Geometry: see drawing. Coordinates: mm, zero at the bounding-box minimum. A direction names the side the tool comes from. Round coordinates to 2 decimals unless told otherwise and drop trailing zeros. Order: outer loops, then holes, each group sorted by start corner. A loop starts at its lowest first (then second) coordinate and runs counter-clockwise, first axis right, second up. Notation, with made-up numbers: (-4.5, -15) - (41.5, -15) arc R19 ccw to (41.5, 15) - close; hole circle Ø5 at (89, -38). An arc over 180 degrees is marked (long way). Put each result on its own line as item: value. Start each with the question number.
1) Access query for the marked faces 1, 2 and 3. Directions: +Z, -Z, +X, -X, +Y, -Y. A direction counts if a zero-diameter tool reaches every point of the face in a straight line with its end or side. Return the directions, or none.
2) Contact query for flat-ended pins moving along their axis: P1, Ø6.5, axis at x = 22, y = 5, coming from the -Z side; P2, Ø4, axis at y = 8.5, z = 12.5, coming from the +X side. Output: stop coordinate, or through.
3) Section A-A on y = 25. Output: boundary loops of the cut face in (x, z).
4) Section B-B on x = 17. Output: boundary loops of the cut face in (y, z), then the cut area to 3 significant figures.
5) Line query: probe 1 along X at (y, z) = (28, 23.5); probe 2 along Y at (x, z) = (40.5, 13); probe 3 along Y at (x, z) = (10, 18.75). Output: solid intervals per line, ascending. Write a range as [from, to].
6) Section C-C on y = 2.5. Output: boundary loops of the cut face in (x, z).
7) Section D-D on x = 10. Output: boundary loops of the cut face in (y, z), then the cut area to 3 significant figures.
8) Mould query, pull axis X, two halves, no side actions, for the marked faces 4, 5 and 6. Classes: +X half, -X half, draft (parallel to the pull), parting line (faces both ways), or undercut.
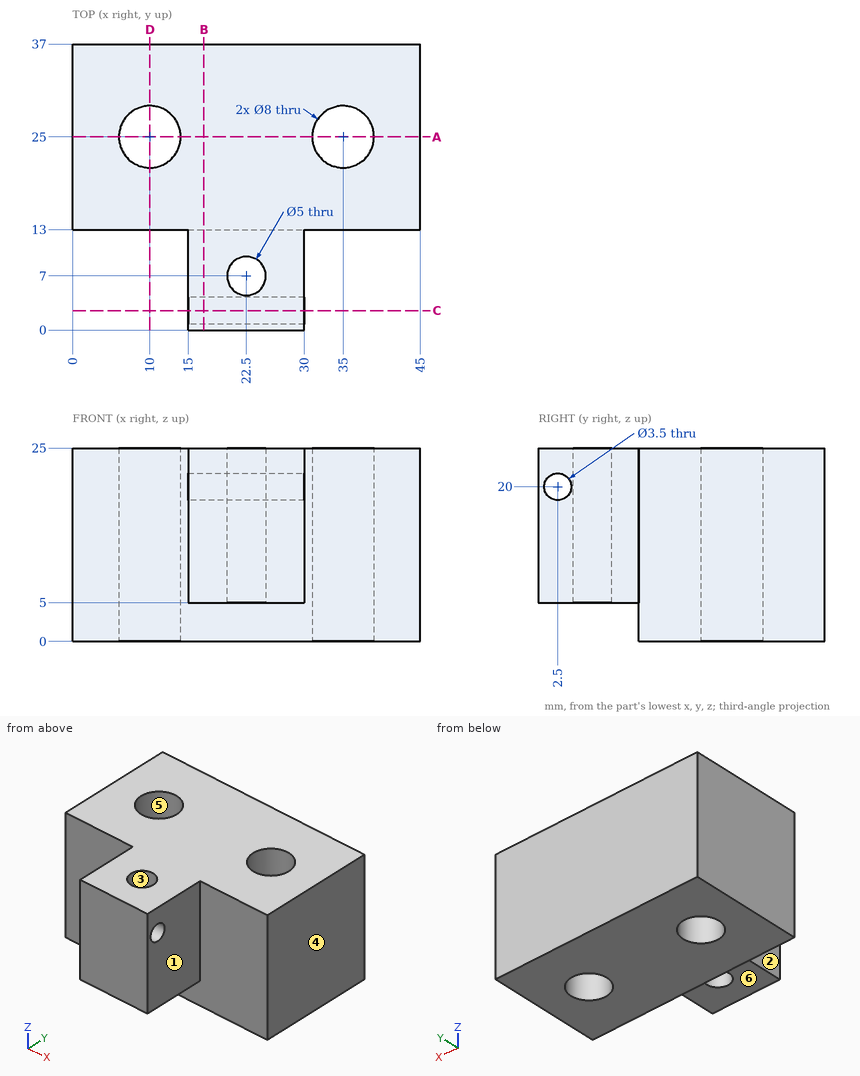
Answer sheet:
1. face 1: +Z, -Z, +X, -Y
1. face 2: +Z, -Z, -X, -Y
1. face 3: +Z, -Z
2. P1: z = 5
2. P2: x = 30
3. outline: (0, 0) - (6, 0) - (6, 25) - (0, 25) - close; (14, 0) - (31, 0) - (31, 25) - (14, 25) - close; (39, 0) - (45, 0) - (45, 25) - (39, 25) - close
4. outline: (0, 5) - (13, 5) - (13, 0) - (37, 0) - (37, 25) - (0, 25) - close; hole circle Ø3.5 at (2.5, 20)
4. area: 850 mm^2
5. probe 1: [0, 7.35], [12.65, 32.35], [37.65, 45]
5. probe 2: [13, 37]
5. probe 3: [13, 21], [29, 37]
6. outline: (15, 5) - (30, 5) - (30, 18.25) - (15, 18.25) - close; (15, 21.75) - (30, 21.75) - (30, 25) - (15, 25) - close
7. outline: (13, 0) - (21, 0) - (21, 25) - (13, 25) - close; (29, 0) - (37, 0) - (37, 25) - (29, 25) - close
7. area: 400 mm^2
8. face 4: +X half
8. face 5: undercut
8. face 6: draft
